```python
from build123d import *

# Parameters (mm, degrees)
MAIN_EXTRUSION_DEPTH = 2000


with BuildPart() as part:
    # Sk Main Extrusion → Main Extrusion (new body)
    with BuildSketch(Plane.XY):
        with BuildLine():
            Line((-3.829999995, 2.532800268), (-11.312491547, 2.92508363))
            ThreePointArc((-11.312491547, 2.92508363), (-11.819968112, 3.366238977), (-11.514692349, 3.965369358))
            Line((-11.514692349, 3.965369358), (-10.100108722, 4.625000536))
            Line((-10.100108722, 4.625000536), (-9.58, 4.300000536))
            Line((-9.58, 4.300000536), (-8.08, 4.300000536))
            Line((-8.08, 4.300000536), (-5.474147193, 5.000000536))
            Line((-5.474147193, 5.000000536), (-4.934147193, 5.000000536))
            Line((-4.934147193, 5.000000536), (-4.23, 4.56))
            Line((-4.23, 4.56), (-4.23, 4.025000268))
            ThreePointArc((-4.23, 4.025000268), (-4.112842712, 3.742157556), (-3.83, 3.625000268))
            Line((-3.83, 3.625000268), (1.67, 3.625000268))
            Line((1.67, 3.625000268), (1.67, 5.120055436))
            Line((1.67, 5.120055436), (1.19886836, 5.120055436))
            ThreePointArc((1.19886836, 5.120055436), (0.3740485, 5.504367422), (0.038, 6.350000268))
            Line((0.038, 6.350000268), (0.038, 6.650000268))
            ThreePointArc((0.038, 6.650000268), (0.3740485, 7.495633114), (1.19886836, 7.8799451))
            Line((1.19886836, 7.8799451), (1.67, 7.8799451))
            Line((1.67, 7.8799451), (1.67, 17.050000268))
            ThreePointArc((1.67, 17.050000268), (1.450330086, 17.580330354), (0.92, 17.800000268))
            Line((0.92, 17.800000268), (0.663, 17.800000268))
            ThreePointArc((0.663, 17.800000268), (0.038, 18.425000268), (0.663, 19.050000268))
            Line((0.663, 19.050000268), (2.17, 19.050000268))
            ThreePointArc((2.17, 19.050000268), (2.700330086, 18.830330354), (2.92, 18.300000268))
            Line((2.92, 18.300000268), (2.92, -17.049999732))
            ThreePointArc((2.92, -17.049999732), (3.139669914, -17.580329818), (3.67, -17.799999732))
            Line((3.67, -17.799999732), (27.295, -17.799999732))
            ThreePointArc((27.295, -17.799999732), (27.92, -18.424999732), (27.295, -19.049999732))
            Line((27.295, -19.049999732), (0.663, -19.049999732))
            ThreePointArc((0.663, -19.049999732), (0.038, -18.424999732), (0.663, -17.799999732))
            Line((0.663, -17.799999732), (0.92, -17.799999732))
            ThreePointArc((0.92, -17.799999732), (1.450330086, -17.580329818), (1.67, -17.049999732))
            Line((1.67, -17.049999732), (1.67, -7.879944832))
            Line((1.67, -7.879944832), (1.19886836, -7.879944832))
            ThreePointArc((1.19886836, -7.879944832), (0.3740485, -7.495632846), (0.038, -6.65))
            Line((0.038, -6.65), (0.038, -6.35))
            ThreePointArc((0.038, -6.35), (0.3740485, -5.504367154), (1.19886836, -5.120055168))
            Line((1.19886836, -5.120055168), (1.67, -5.120055168))
            Line((1.67, -5.120055168), (1.67, -3.625))
            Line((1.67, -3.625), (-3.83, -3.625))
            ThreePointArc((-3.83, -3.625), (-4.112842712, -3.742157288), (-4.23, -4.025))
            Line((-4.23, -4.025), (-4.23, -4.56))
            Line((-4.23, -4.56), (-4.934147193, -5))
            Line((-4.934147193, -5), (-5.474147193, -5))
            Line((-5.474147193, -5), (-8.08, -4.3))
            Line((-8.08, -4.3), (-9.58, -4.3))
            Line((-9.58, -4.3), (-10.100108722, -4.625))
            Line((-10.100108722, -4.625), (-11.51469235, -3.965368821))
            ThreePointArc((-11.51469235, -3.965368821), (-11.819968112, -3.36623844), (-11.312491547, -2.925083093))
            Line((-11.312491547, -2.925083093), (-3.830000005, -2.532799732))
            Line((-3.830000005, -2.532799732), (1.67, -2.436796875))
            Line((1.67, -2.436796875), (1.67, 2.436797411))
            Line((1.67, 2.436797411), (-3.829999995, 2.532800268))
        make_face()
    extrude(amount=-MAIN_EXTRUSION_DEPTH)


solid = part.part
```
Geometry: final body of the model. Coordinates: model frame, mm. A direction names the side the tool comes from. Round coordinates to 2 decimals unless told otherwise and drop trailing zeros. Loops run counter-clockwise (first coordinate to the right, second up) from the corner with the lowest first, then second, coordinate; pieces in that order, holes last. Notation, with made-up numbers: (-38, -38) -> (-11, -38) arc R5 ccw to (-11, -30) -> close; hole circle Ø3 at (-29, 48.25). An arc over 180 degrees is marked (long way). Use one line per item in the form item = value.
Item 1: Contact query for flat-ended pins moving along their axis: pin 1 Ø10 at (y, z) = (8.5, -1684) entering from +X; pin 2 Ø3 at (x, z) = (-2, -1428) entering from -Y (3 decimals); pin 3 Ø2.5 at (y, z) = (-0.5, -1070.5) entering from -X. Output: stop coordinate, or through.
Evaluation:
pin_1 = 2.92
pin_2 = -3.625
pin_3 = 1.67
Item 2: Cut plane A-A on x = 18. Output: boundary loops of the cut face in (y, z).
Evaluation:
outline = (-19.05, -2000) -> (-17.8, -2000) -> (-17.8, 0) -> (-19.05, 0) -> close
Item 3: Material intervals for probe 1 along Y at (x, z) = (-6, -558); probe 2 along Y at (x, z) = (-7, -194.5); probe 3 along X at (y, z) = (-16.5, -1799), sorted ascending.
Evaluation:
probe_1 = -4.86 to -2.65, 2.65 to 4.86
probe_2 = -4.59 to -2.7, 2.7 to 4.59
probe_3 = 1.67 to 2.92
Item 4: Access query for faces 1 (the flat face through (2.92, 1, -986)), 2 (the flat face through (2, -4, -2000)). Directions: +Z, -Z, +X, -X, +Y, -Y. A direction counts if a zero-diameter tool reaches every point of the face in a straight line with its end or side. Return the directions, or none.
Evaluation:
face_1 = +Z, -Z, +X, +Y
face_2 = -Z, +X, -X, +Y, -Y
